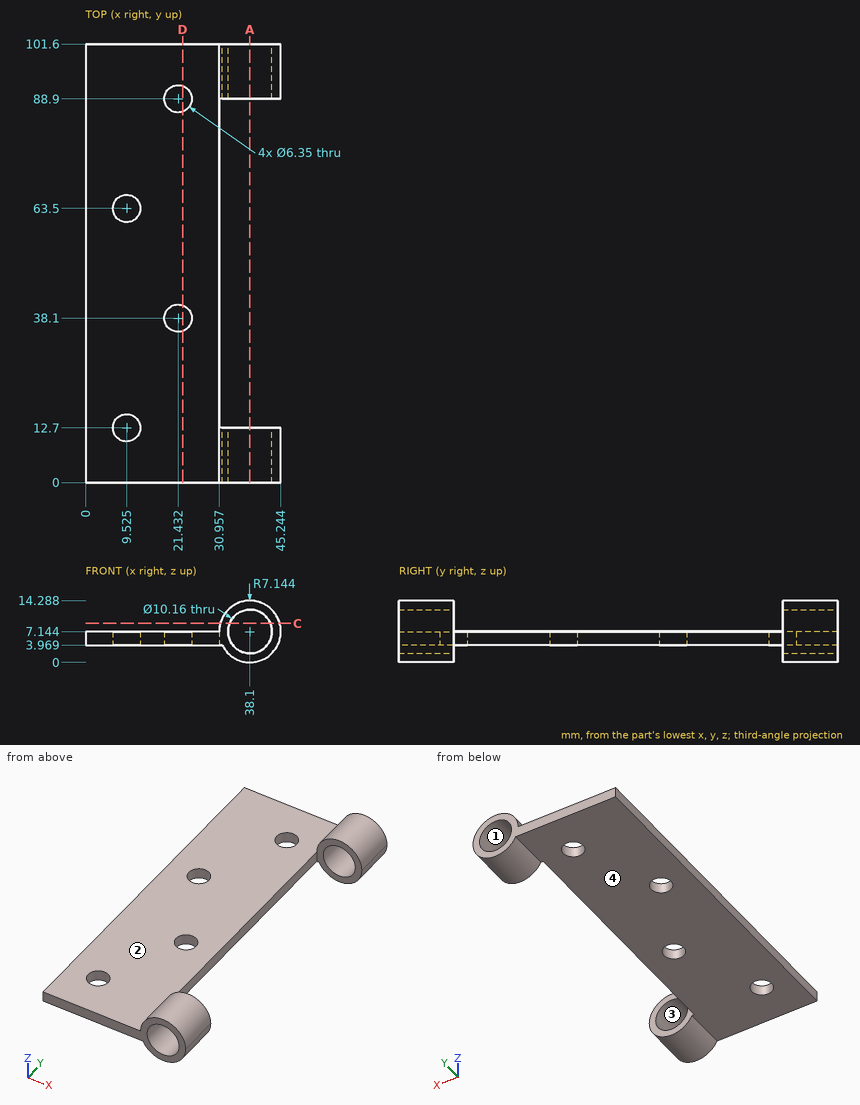
Study the drawing (mm; zero at the part's minimum x, y, z) and answer. A direction names the side the tool comes from. Round coordinates to 2 decimals unless told otherwise and drop trailing zeros. Write each loop counter-clockwise with the first axis right and the second up, starting at its lowest first coordinate (ties: lowest second). Pieces come first, ordered by that corner, then holes. Notation, with made-up numbers: (48, -23.75) -> (94, -23.75) arc R26 ccw to (94, 0.25) -> close; hole circle Ø1 at (-18, 87). An arc over 180 degrees is marked (long way). Use CSV: the item, a comma, the result in double quotes. Start each with the question number.
(1) Consider L1, parallel to Y at x = 8.5, z = 6.5 (1 decimal); L2, parallel to Y at x = 12, z = 4.75; L3, parallel to Z at x = 2.5, y = 91. Determine where each line is inside the solid, lowest interval first. Write a range as from..to.
(2) Section A-A on x = 38.1 is taken. Give the vertices of the cut face in (y, z).
(3) Each of these flat-tipped pins is pushed along its axis until it touches: pin 1 (4 mm diameter, centred on y = 53, z = 3, fed in from +X); pin 2 (8.5 mm diameter, centred on x = 21.43, y = 38.1, fed in from +Z); pin 3 (7 mm diameter, centred on x = 36, z = 9, fed in from -Y); pin 4 (10 mm diameter, centred on x = 9.525, y = 12.7, fed in from -Z). Where does it stop, or does it pass through?
(4) Section C-C on z = 9 is taken. Give the vertices of the cut face in (x, y), then the cut area to 3 significant figures.
(5) The mould has two halves that part along X. Classify the marked faces 1 and 2: released by +X, released by -X, zero draft, split by the parting line, or undercut.
(6) Which of the six approach directions +Z, -Z, +X, -X, +Y, -Y give full straight-line access (tool end or side, diameter ignored) to the marked faces 3 and 4?
(7) Section D-D on x = 22.5 is taken. Give the vertices of the cut face in (y, z).
A:
1,L1,"y = 0..9.7, 15.7..60.5, 66.5..101.6"
1,L2,"y = 0..10.71, 14.69..61.51, 65.49..101.6"
1,L3,"z = 3.97..7.14"
2,outline,"(0, 0) -> (12.7, 0) -> (12.7, 2.06) -> (0, 2.06) -> close; (0, 12.22) -> (12.7, 12.22) -> (12.7, 14.29) -> (0, 14.29) -> close; (88.9, 0) -> (101.6, 0) -> (101.6, 2.06) -> (88.9, 2.06) -> close; (88.9, 12.22) -> (101.6, 12.22) -> (101.6, 14.29) -> (88.9, 14.29) -> close"
3,pin 1,"stops at x = 30.96"
3,pin 2,"stops at z = 7.14"
3,pin 3,"stops at y = 0"
3,pin 4,"stops at z = 3.97"
4,outline,"(31.2, 0) -> (33.37, 0) -> (33.37, 12.7) -> (31.2, 12.7) -> close; (31.2, 88.9) -> (33.37, 88.9) -> (33.37, 101.6) -> (31.2, 101.6) -> close; (42.83, 0) -> (45, 0) -> (45, 12.7) -> (42.83, 12.7) -> close; (42.83, 88.9) -> (45, 88.9) -> (45, 101.6) -> (42.83, 101.6) -> close"
4,area,"110 mm²"
5,face 1,"undercut"
5,face 2,"zero draft"
6,face 3,"+Y, -Y"
6,face 4,"-Z, -X, +Y, -Y"
7,outline,"(0, 3.97) -> (35.11, 3.97) -> (35.11, 7.14) -> (0, 7.14) -> close; (41.09, 3.97) -> (85.91, 3.97) -> (85.91, 7.14) -> (41.09, 7.14) -> close; (91.89, 3.97) -> (101.6, 3.97) -> (101.6, 7.14) -> (91.89, 7.14) -> close"
